from build123d import *

# Parameters (mm, degrees)
F0_W      = 29
F0_H      = 9
F1_DEPTH  = 27
F0_W_2    = 8
F0_R      = 1.6
F2_DEPTH  = 2
F3_W      = 15
F3_H      = 11.7
F3_R      = 1.5
F4_DEPTH  = 10
F5_DEPTH  = 6
F6_DEPTH  = 7.5
F7_R      = 2.5
F8_R      = 3
F10_DEPTH = 2
F11_DEPTH = 3


# Not quite as in the source:
# - a feature names something its author has since deleted; it is built from what else it names


with BuildPart() as f1:
    # F0 (on Top) → F1 (new body)
    with BuildSketch(Plane.XY):
        with Locations((3.6698216572, -1.1730009172)):
            Rectangle(F0_W, F0_H)
    extrude(amount=F1_DEPTH)

    # F0 (on Top) → F2 (join)
    with BuildSketch(Plane.XY):
        with Locations((-14.8301783428, -1.1730009172)):
            Rectangle(F0_W_2, F0_H)
        with Locations((-14.3301783428, -1.1730009172)):
            Circle(F0_R, mode=Mode.SUBTRACT)
        with Locations((22.1698216572, -1.1730009172)):
            Rectangle(F0_W_2, F0_H)
        with Locations((21.6698216572, -1.1730009172)):
            Circle(F0_R, mode=Mode.SUBTRACT)
    extrude(amount=F2_DEPTH)

    # F3 (on face) → F4 (cut)
    with BuildSketch(Plane.XZ.offset(5.6730009172)):
        with Locations((-0.1801783428, 17.9)):
            Rectangle(F3_W, F3_H)
        with Locations((13.3198216572, 17.8843773901)):
            Circle(F3_R)
    extrude(amount=-F4_DEPTH, mode=Mode.SUBTRACT)

    # F3 (on face) → F5 (cut)
    with BuildSketch(Plane.XZ.offset(5.6730009172)):
        with BuildLine():
            Line((15.0198216572, 23.75), (7.3198216572, 23.75))
            Line((7.3198216572, 23.75), (7.3198216572, 12.05))
            Line((7.3198216572, 12.05), (15.0198216572, 12.05))
            Line((15.0198216572, 12.05), (15.0198216572, 15.4125359713))
            ThreePointArc((15.0198216572, 15.4125359713), (10.3198216572, 17.8843773901), (15.0198216572, 20.356218809))
            Line((15.0198216572, 20.356218809), (15.0198216572, 23.75))
        make_face()
    extrude(amount=-F5_DEPTH, mode=Mode.SUBTRACT)

    # F3 (on face) → F6 (cut)
    with BuildSketch(Plane.XZ.offset(5.6730009172)):
        with BuildLine():
            ThreePointArc((16.3198216572, 17.8843773901), (15.9750052667, 19.2808013945), (15.0198216572, 20.356218809))
            Line((15.0198216572, 20.356218809), (15.0198216572, 15.4125359713))
            ThreePointArc((15.0198216572, 15.4125359713), (15.9750052667, 16.4879533858), (16.3198216572, 17.8843773901))
        make_face()
        with BuildLine():
            Line((15.0198216572, 15.4125359713), (15.0198216572, 20.356218809))
            ThreePointArc((15.0198216572, 20.356218809), (10.3198216572, 17.8843773901), (15.0198216572, 15.4125359713))
        make_face()
        with Locations((13.3198216572, 17.8843773901)):
            Circle(F3_R, mode=Mode.SUBTRACT)
    extrude(amount=-F6_DEPTH, mode=Mode.SUBTRACT)

    # F7
    f7_edges = [f1.edges().sort_by_distance(p)[0] for p in [
        (-10.830178, -1.173001, 27),
        (18.169822, -1.173001, 27),
    ]]
    fillet(f7_edges, radius=F7_R)

    # F8
    f8_edges = [f1.edges().sort_by_distance(p)[0] for p in [
        (-18.830178, 3.326999, 1),
        (-18.830178, -5.673001, 1),
        (26.169822, -5.673001, 1),
        (26.169822, 3.326999, 1),
    ]]
    fillet(f8_edges, radius=F8_R)

    # F9 (on face) → F10 (join)
    with BuildSketch(Plane.XZ.offset(5.6730009172)):
        with BuildLine():
            Line((-14.0801783428, 12.05), (-10.8301783428, 12.05))
            Line((-10.8301783428, 12.05), (-10.8301783428, 16.9))
            ThreePointArc((-10.8301783428, 16.9), (-11.8301783428, 17.9), (-10.8301783428, 18.9))
            Line((-10.8301783428, 18.9), (-10.8301783428, 23.75))
            Line((-10.8301783428, 23.75), (-14.0801783428, 23.75))
            Line((-14.0801783428, 23.75), (-14.0801783428, 12.05))
        make_face()
        with BuildLine():
            Line((18.1698216572, 16.9), (18.1698216572, 12.05))
            Line((18.1698216572, 12.05), (21.4198216572, 12.05))
            Line((21.4198216572, 12.05), (21.4198216572, 23.75))
            Line((21.4198216572, 23.75), (18.1698216572, 23.75))
            Line((18.1698216572, 23.75), (18.1698216572, 18.9))
            ThreePointArc((18.1698216572, 18.9), (18.8769284384, 18.6071067812), (19.1698216572, 17.9))
            ThreePointArc((19.1698216572, 17.9), (18.8769284384, 17.1928932188), (18.1698216572, 16.9))
        make_face()
    extrude(amount=-F10_DEPTH)

    # F9 (on face) → F11 (cut)
    with BuildSketch(Plane.XZ.offset(5.6730009172)):
        with BuildLine():
            Line((-10.8301783428, 18.9), (-10.8301783428, 16.9))
            ThreePointArc((-10.8301783428, 16.9), (-10.1230715616, 17.1928932188), (-9.8301783428, 17.9))
            ThreePointArc((-9.8301783428, 17.9), (-10.1230715616, 18.6071067812), (-10.8301783428, 18.9))
        make_face()
        with BuildLine():
            ThreePointArc((18.1698216572, 18.9), (17.1698216572, 17.9), (18.1698216572, 16.9))
            Line((18.1698216572, 16.9), (18.1698216572, 18.9))
        make_face()
    extrude(amount=-F11_DEPTH, mode=Mode.SUBTRACT)


solid = f1.part
The model under review builds one solid part; all positions refer to its coordinate system, in mm. A direction names the side the tool comes from. Coordinates: 2 decimals unless noted, no trailing zeros. Write each loop counter-clockwise with the first axis right and the second up, starting at its lowest first coordinate (ties: lowest second). Pieces come first, ordered by that corner, then holes. Notation, with made-up numbers: (9.5, 74) - (22.5, 74) arc R16 cw to (22.5, 100) - close; hole circle Ø1 at (1.5, 12). An arc over 180 degrees is marked (long way). Answer as a JSON object with one key per item and string values. Group by question number.
1. Add section D-D (z = 4). Give the boundary of the cut face in (x, y), plus the area to 3 significant figures.
2. Add section A-A (x = -6). Give the boundary of the cut face in (y, z).
3. To check wall thickness, follow probe 1 along X at (y, z) = (-1.25, 1.5); probe 2 along Z at (x, y) = (6, -2.25); probe 3 along Z at (x, y) = (-12.5, -4.5). State the ranges of each line that lie inside material, in increasing order.
4. Add section B-B (y = -0.25). Give the boundary of the cut face in (x, z).
5. Mouldability with a two-part tool opening along Z and no side actions: class faces 1 (the face through (18, -2.673, 18)), 2 (the face through (4, -1, 27)), 3 (the face through (-7.68, -1, 18)), 4 (the face through (-12.8, -0.7, 1)) as pulls with the +Z half, pulls with the -Z half, needs draft (parallel to the pull), parting line crosses it, or undercut.
6. Clearance check with flat-ended pins moving along their axes: pin 1 Ø0.6 at (x, y) = (19.5, -5) entering from +Z; pin 2 Ø1 at (y, z) = (-4.5, 18) entering from +X; pin 3 Ø5 at (y, z) = (-1.5, 18.5) entering from -X; pin 4 Ø1.9 at (x, y) = (21.67, -1.17) entering from +Z. State where each tip first meets the part, or that it passes through.
7. Machinability: for faces 5 (the face through (4, -1, 23.75)), 6 (the face through (-14.08, -5, 18)), 7 (the face through (20, -3.673, 18)), 8 (the face through (7.32, 2, 18)), 9 (the face through (20, -5, 12.05)), which of the approach directions +Z, -Z, +X, -X, +Y, -Y give a long, thin tool a straight path to every point of the face, cutting with its end or side? Answer none if there is none.
8. Add section C-C (y = -4.25). Give the boundary of the cut face in (x, z), plus the area to 3 significant figures.
Findings:
{
 "1": {"outline": "(-10.83, -5.67) - (18.17, -5.67) - (18.17, 3.33) - (-10.83, 3.33) - close", "area": "261 mm²"},
 "2": {"outline": "(-5.67, 0) - (3.33, 0) - (3.33, 12.05) - (-5.67, 12.05) - close; (-5.67, 23.75) - (3.33, 23.75) - (3.33, 27) - (-5.67, 27) - close"},
 "3": {"probe 1": "-18.83 to -15.93, -12.73 to 20.07, 23.27 to 26.17", "probe 2": "0 to 12.05, 23.75 to 27", "probe 3": "0 to 2, 12.05 to 23.75"},
 "4": {"outline": "(-18.83, 0) - (-15.64, 0) - (-15.64, 2) - (-18.83, 2) - close; (-13.02, 0) - (20.36, 0) - (20.36, 2) - (18.17, 2) - (18.17, 24.5) arc R2.5 ccw to (15.67, 27) - (-8.33, 27) arc R2.5 ccw to (-10.83, 24.5) - (-10.83, 2) - (-13.02, 2) - close; (22.98, 0) - (26.17, 0) - (26.17, 2) - (22.98, 2) - close; hole (-7.68, 12.05) - (15.02, 12.05) - (15.02, 15.41) arc R3 ccw to (15.02, 20.36) - (15.02, 23.75) - (-7.68, 23.75) - close"},
 "5": {"face 1": "undercut", "face 2": "pulls with the +Z half", "face 3": "undercut", "face 4": "needs draft"},
 "6": {"pin 1": "z = 23.75", "pin 2": "x = 21.42", "pin 3": "x = -14.08", "pin 4": "through"},
 "7": {"face 5": "-Y", "face 6": "+Z, -X, +Y, -Y", "face 7": "+Z, +X, +Y", "face 8": "+Y, -Y", "face 9": "+X, +Y, -Y"},
 "8": {"outline": "(-18.38, 0) - (25.72, 0) - (25.72, 2) - (18.17, 2) - (18.17, 12.05) - (21.42, 12.05) - (21.42, 23.75) - (18.17, 23.75) - (18.17, 24.5) arc R2.5 ccw to (15.67, 27) - (-8.33, 27) arc R2.5 ccw to (-10.83, 24.5) - (-10.83, 23.75) - (-14.08, 23.75) - (-14.08, 12.05) - (-10.83, 12.05) - (-10.83, 2) - (-18.38, 2) - close; hole circle Ø2 at (-10.83, 17.9); hole (-7.68, 12.05) - (15.02, 12.05) - (15.02, 15.41) arc R3 ccw to (15.02, 20.36) - (15.02, 23.75) - (-7.68, 23.75) - close; hole circle Ø2 at (18.17, 17.9)", "area": "610 mm²"}
}
